Verification items for the finished model (mm, model axes). A direction names the side the tool comes from. Round coordinates to 2 decimals unless told otherwise and drop trailing zeros. Order: outer loops, then holes, each group sorted by start corner. A loop starts at its lowest first (then second) coordinate and runs counter-clockwise, first axis right, second up. Notation, with made-up numbers: (46.25, 82.25) -> (65.25, 82.25) arc R32 ccw to (65.25, 117.25) -> close; hole circle Ø4 at (-12.75, 52). An arc over 180 degrees is marked (long way). Return JSON: item names as keys, results as strings. Group by question number.
Item 1: Draft check along Y on faces 1 (the cylindrical face through (7.86, -23.6, 5.07)), 2 (the flat face through (20, -34, 10)), 3 (the cylindrical face through (20.1, -6.4, 8.2)). Enter one of: pulls with the +Y half, pulls with the -Y half, needs draft (parallel to the pull), parting line crosses it, or undercut.
Item 2: Sectioned sample at D-D on y = -43. Record the cut outline in (x, z), plus the area to 3 significant figures.
Item 3: Depth check by flat-ended pin: pin 1 Ø6 at (x, z) = (34, 1.5) entering from -Y; pin 2 Ø0.8 at (y, z) = (-1, 8.5) entering from -X; pin 3 Ø1 at (x, y) = (16, -37) entering from +Z. Enter the tip coordinate at first touch or a pass-through.
Item 4: Scan lines: probe 1 along Y at (x, z) = (20, 3.5); probe 2 along Y at (x, z) = (26, 1.5); probe 3 along Y at (x, z) = (17, 2.5). Record each from-to range of solid material in increasing order. Write a range as from..to.
Item 5: Access from +Z, -Z, +X, -X, +Y, -Y to the whole of each face (thin tool, end or side, straight path). Record for faces 4 (the flat face through (34.9, -2, 8)), 5 (the cylindrical face through (32.14, -23.6, 5.07)), 6 (the flat face through (23, -63, 1)).
Item 6: Sectioned sample at B-B on y = -20.5. Record the cut outline in (x, z), plus the area to 3 significant figures.
Item 7: Sectioned sample at A-A on z = 2.25. Give the number of separate pieces and of enclosed holes in the cut face, plus the area to 3 significant figures.
```python
from build123d import *

# Parameters (mm, degrees)
SKETCH_1_W          = 40
SKETCH_1_H          = 70.5
EXTRUDE_1_DEPTH     = 10
SKETCH_2_R          = 14.25
CUT_EXTRUDE_1_DEPTH = 12
SKETCH_3_R          = 15.05
CUT_EXTRUDE_2_DEPTH = 1.1
CHAMFER_1_SIZE      = 2
FILLET_1_R          = 20
SKETCH_4_R          = 1.5
CUT_EXTRUDE_3_DEPTH = 15
SKETCH_5_W          = 26
SKETCH_5_H          = 15
CUT_EXTRUDE_4_DEPTH = 15
FILLET_2_R          = 3
EXTRUDE_START       = -1
SKETCH_7_R          = 14.25
SKETCH_7_R_2        = 13
EXTRUDE_2_DEPTH     = 1
CUT_EXTRUDE_5_DEPTH = 3.2
CHAMFER_2_SIZE      = 0.5


with BuildPart() as part:
    # 草图1 → 凸台-拉伸1 (new body)
    with BuildSketch(Plane.XY):
        with Locations((20, -34.75)):
            Rectangle(SKETCH_1_W, SKETCH_1_H)
    extrude(amount=EXTRUDE_1_DEPTH)

    # 草图2 → 切除-拉伸1 (cut)
    with BuildSketch(Plane.XY.offset(10)):
        with Locations((20, -50)):
            Circle(SKETCH_2_R)
    extrude(amount=-CUT_EXTRUDE_1_DEPTH, mode=Mode.SUBTRACT)

    # 草图3 → 切除-拉伸2 (cut)
    with BuildSketch(Plane(origin=(0, 0, 8), x_dir=(-1, 0, 0), z_dir=(0, 0, -1))):
        with Locations((-20, -50)):
            Circle(SKETCH_3_R)
    extrude(amount=-CUT_EXTRUDE_2_DEPTH, mode=Mode.SUBTRACT)

    # 倒角1
    chamfer_1_edges = [part.edges().sort_by_distance(p)[0] for p in [
        (0, 0.5, 5),
        (40, 0.5, 5),
    ]]
    chamfer(chamfer_1_edges, length=CHAMFER_1_SIZE)

    # 圆角1
    fillet_1_edges = [part.edges().sort_by_distance(p)[0] for p in [
        (0, -70, 5),
        (40, -70, 5),
    ]]
    fillet(fillet_1_edges, radius=FILLET_1_R - 0.0001)  # a hair under: the kernel refuses the full size

    # 草图4 → 切除-拉伸3 (cut)
    with BuildSketch(Plane(origin=(0, 0, 0), x_dir=(-1, 0, 0), z_dir=(0, 0, -1))):
        with Locations((-32, -3.5)):
            Circle(SKETCH_4_R)
        with Locations((-20, -3.5)):
            Circle(SKETCH_4_R)
        with Locations((-8, -3.5)):
            Circle(SKETCH_4_R)
    extrude(amount=-CUT_EXTRUDE_3_DEPTH, mode=Mode.SUBTRACT)

    # 草图5 → 切除-拉伸4 (cut)
    with BuildSketch(Plane(origin=(0, 0, 0), x_dir=(-1, 0, 0), z_dir=(0, 0, -1))):
        with Locations((-20, -17)):
            Rectangle(SKETCH_5_W, SKETCH_5_H)
    extrude(amount=-CUT_EXTRUDE_4_DEPTH, mode=Mode.SUBTRACT)

    # 圆角2
    fillet_2_edges = [part.edges().sort_by_distance(p)[0] for p in [
        (7, -9.5, 5),
        (7, -24.5, 5),
        (33, -24.5, 5),
        (33, -9.5, 5),
    ]]
    fillet(fillet_2_edges, radius=FILLET_2_R)

    # 草图7 → 凸台-拉伸2 (add)
    with BuildSketch(Plane(origin=(0, 0, 0), x_dir=(-1, 0, 0), z_dir=(0, 0, -1)).offset(EXTRUDE_START)):
        with Locations((-20, -50)):
            Circle(SKETCH_7_R)
        with Locations((-20, -50)):
            Circle(SKETCH_7_R_2, mode=Mode.SUBTRACT)
    extrude(amount=EXTRUDE_2_DEPTH)

    # 草图8 → 切除-拉伸5 (cut)
    with BuildSketch(Plane.XY.offset(10)):
        with BuildLine():
            Line((5.1, -3.5), (5.1, 0.5))
            Line((5.1, 0.5), (10.9, 0.5))
            Line((10.9, 0.5), (10.9, -3.5))
            ThreePointArc((10.9, -3.5), (8, -6.4), (5.1, -3.5))
        make_face()
        with BuildLine():
            Line((17.1, -3.5), (17.1, 0.5))
            Line((17.1, 0.5), (22.9, 0.5))
            Line((22.9, 0.5), (22.9, -3.5))
            ThreePointArc((22.9, -3.5), (20, -6.4), (17.1, -3.5))
        make_face()
        with BuildLine():
            Line((34.9, -3.5), (34.9, 0.5))
            Line((34.9, 0.5), (29.1, 0.5))
            Line((29.1, 0.5), (29.1, -3.5))
            ThreePointArc((29.1, -3.5), (32, -6.4), (34.9, -3.5))
        make_face()
    extrude(amount=-CUT_EXTRUDE_5_DEPTH, mode=Mode.SUBTRACT)

    # 倒角2
    chamfer_2_edges = [part.edges().sort_by_distance(p)[0] for p in [
        (8, -6.4, 10),
        (10.9, -1.5, 10),
        (5.1, -1.5, 10),
        (32, -6.4, 10),
        (34.9, -1.5, 10),
        (29.1, -1.5, 10),
        (20, -6.4, 10),
        (22.9, -1.5, 10),
        (17.1, -1.5, 10),
    ]]
    chamfer(chamfer_2_edges, length=CHAMFER_2_SIZE)


solid = part.part
```
Recorded:
{
 "1": {"face 1": "undercut", "face 2": "needs draft", "face 3": "pulls with the +Y half"},
 "2": {"outline": "(0, 0) -> (9.05, 0) -> (9.05, 1) -> (7.59, 1) -> (7.59, 8) -> (6.68, 8) -> (6.68, 9.1) -> (7.59, 9.1) -> (7.59, 10) -> (0, 10) -> close; (30.95, 0) -> (40, 0) -> (40, 10) -> (32.41, 10) -> (32.41, 9.1) -> (33.32, 9.1) -> (33.32, 8) -> (32.41, 8) -> (32.41, 1) -> (30.95, 1) -> close", "area": "153 mm²"},
 "3": {"pin 1": "y = -66.7", "pin 2": "x = 0.1", "pin 3": "z = 1"},
 "4": {"probe 1": "-70..-64.25, -35.75..-24.5, -9.5..-5, -2..0.5", "probe 2": "-69.08..-62.93, -37.07..-24.5, -9.5..0.5", "probe 3": "-69.77..-63.93, -36.07..-24.5, -9.5..0.5"},
 "5": {"face 4": "+Z, +Y", "face 5": "+Z, -Z", "face 6": "+Z"},
 "6": {"outline": "(0, 0) -> (7, 0) -> (7, 10) -> (0, 10) -> close; (33, 0) -> (40, 0) -> (40, 10) -> (33, 10) -> close", "area": "140 mm²"},
 "7": {"separate pieces": "1", "enclosed holes": "5", "area": "1,600 mm²"}
}
